Check sheet for the drawn part. Datum: minimum x, y, z corner. Units: mm. A direction names the side the tool comes from. Coordinates: 2 decimals unless noted, no trailing zeros. Order: outer loops, then holes, each group sorted by start corner. A loop starts at its lowest first (then second) coordinate and runs counter-clockwise, first axis right, second up. Notation, with made-up numbers: (67, 80.5) - (77, 80.5) arc R23 cw to (77, 110.5) - close; hole circle Ø2 at (4.25, -25). An arc over 180 degrees is marked (long way). Put each result on its own line as item: value.
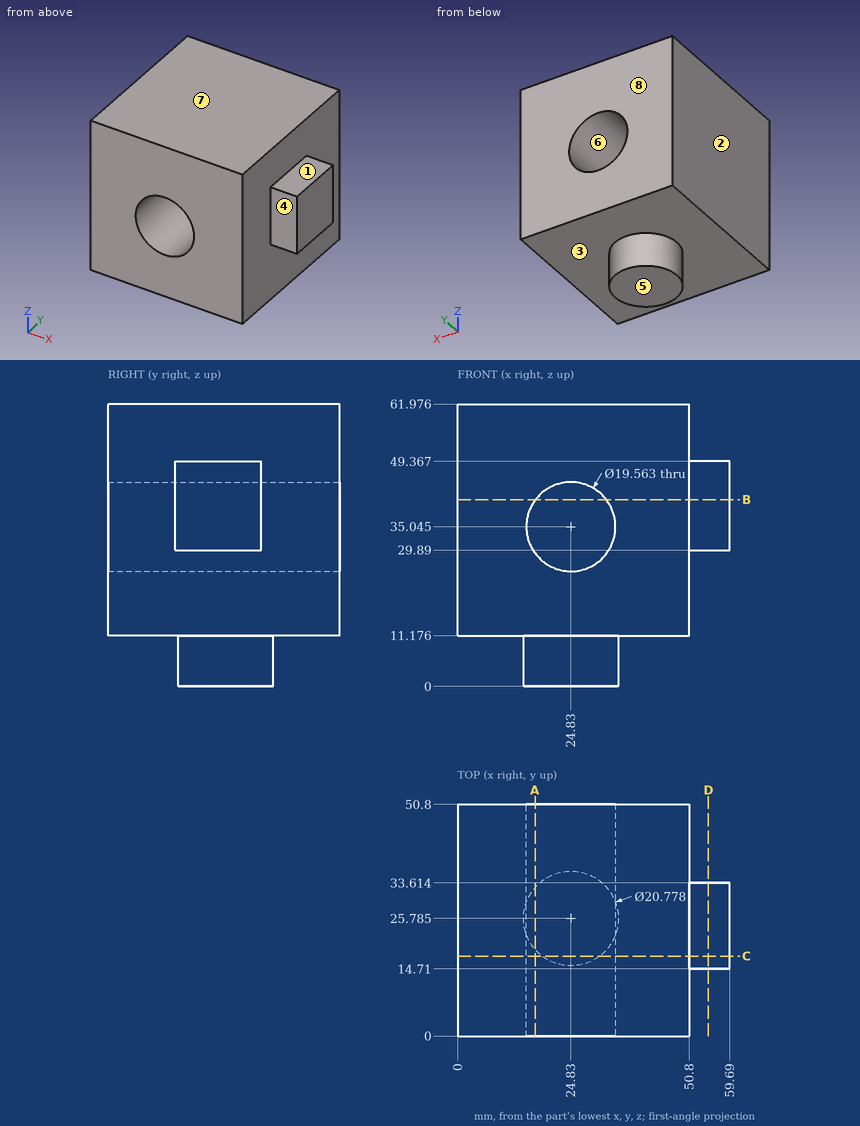
Q1. Section check B-B on z = 41. Record the boundary of the cut face in (x, y).
Answer block:
outline: (0, 0) - (17.07, 0) - (17.07, 50.8) - (0, 50.8) - close; (32.59, 0) - (50.8, 0) - (50.8, 14.71) - (59.69, 14.71) - (59.69, 33.61) - (50.8, 33.61) - (50.8, 50.8) - (32.59, 50.8) - close
Q2. Section check D-D on x = 55. Record the boundary of the cut face in (y, z), then the cut area to 3 significant figures.
Answer block:
outline: (14.71, 29.89) - (33.61, 29.89) - (33.61, 49.37) - (14.71, 49.37) - close
area: 368 mm^2
Q3. Depth check by flat-ended pin: pin 1 Ø4.5 at (x, y) = (56.5, 20.5) entering from -Z; pin 2 Ø7 at (x, y) = (56.5, 19.5) entering from +Z; pin 3 Ø2 at (x, z) = (37, 9.5) entering from -Y; pin 4 Ø7 at (x, z) = (55.5, 38) entering from -Y. Enter the tip coordinate at first touch or a pass-through.
Answer block:
pin 1: stops at z = 29.89
pin 2: stops at z = 49.37
pin 3: passes through
pin 4: stops at y = 14.71
Q4. Draft check along Z on the marked faces 5, 6, 7 and 8. Enter one of: pulls with the +Z half, pulls with the -Z half, needs draft (parallel to the pull), parting line crosses it, or undercut.
Answer block:
face 5: pulls with the -Z half
face 6: undercut
face 7: pulls with the +Z half
face 8: needs draft
Q5. Access from +Z, -Z, +X, -X, +Y, -Y to the whole of each face (thin tool, end or side, straight path). Record for the marked faces 1, 2, 3 and 4.
Answer block:
face 1: +Z, +X, +Y, -Y
face 2: +Z, -Z, -X, +Y, -Y
face 3: -Z
face 4: +Z, -Z, +X, -Y
Q6. Section check A-A on x = 17. Record the boundary of the cut face in (y, z).
Answer block:
outline: (0, 11.18) - (18.96, 11.18) - (18.96, 0) - (32.61, 0) - (32.61, 11.18) - (50.8, 11.18) - (50.8, 29.18) - (0, 29.18) - close; (0, 40.91) - (50.8, 40.91) - (50.8, 61.98) - (0, 61.98) - close
Q7. Thickness scan on L1, parallel to Z at x = 11, y = 32; L2, parallel to X at y = 6.5, z = 21; L3, parallel to Z at x = 28.5, y = 36 (1 decimal). Record the ranges inside material, lowest first. Write a range as [from, to].
Answer block:
L1: z = [11.18, 61.98]
L2: x = [0, 50.8]
L3: z = [11.2, 26], [44.1, 62]
Q8. Section check C-C on y = 17.5. Record the boundary of the cut face in (x, z) (1 decimal).
Answer block:
outline: (0, 11.2) - (18.6, 11.2) - (18.6, 0) - (31.1, 0) - (31.1, 11.2) - (50.8, 11.2) - (50.8, 29.9) - (59.7, 29.9) - (59.7, 49.4) - (50.8, 49.4) - (50.8, 62) - (0, 62) - close; hole circle Ø19.6 at (24.8, 35)
